Geometry check sheet. Reference: the model listing, model coordinates, mm. A direction names the side the tool comes from. Coordinates: 2 decimals unless noted, no trailing zeros. Loops run counter-clockwise (first coordinate to the right, second up) from the corner with the lowest first, then second, coordinate; pieces in that order, holes last. Notation, with made-up numbers: M -30.5,28 L 19.5,28 A29 cw 19.5,56 Z; hole C 44.25,-31 d7. An arc over 180 degrees is marked long. Use CSV: the item, a comma, the result in double quotes.
Autodesk Inventor part; units mm, degrees
ref_plane "YZ Plane" through (0, 0, 0) normal (1, 0, 0) x (0, 1, 0)
ref_plane "XZ Plane" through (0, 0, 0) normal (0, 1, 0) x (-1, 0, 0)
sketch "Sketch1" plane through (0, 0, 0) normal (1, 0, 0) x (0, 1, 0)
  line L0 (-5, 130) -> (-5, -130)
  line L1 (-5, -130) -> (5, -130)
  line L2 (5, -130) -> (5, 130)
  line L3 (5, 130) -> (-5, 130)
  line L4 (-5, 130) -> (5, -130) construction
  line L5 (-5, -130) -> (5, 130) construction
  circle A0 centre (0, -124) radius 1.95
  circle A1 centre (0, 124) radius 1.95
  line L6 (-5, -70) -> (-5, -60)
  circle A2 centre (0, -65) radius 1.5
  circle A3 centre (0, 65) radius 1.5
  point P0 (0, 0)
  point P1 (0, 0)
  dimension "d0" = 260
  dimension "d1" = 10
  dimension "d2" = 3.9
  dimension "d3" = 6
  dimension "d4" = 3.9
  dimension "d5" = 6
  dimension "d25" = 3
  dimension "d27" = 59
  dimension "d28" = 3
  dimension "d29" = 59
extrude "Extrusion1" add sketch "Sketch1" along normal blind 5
fillet "Fillet1" radius 2 4 edges at (2.5, 5, 130) (2.5, -5, 130) (2.5, 5, -130) (2.5, -5, -130)
sketch "Sketch2" plane through (5, 0, 0) normal (1, 0, 0) x (0, 0, -1)
  line L0 (-128, -5) -> (128, -5)
  line L1 (60, -5) -> (70, -5)
  line L2 (70, -5) -> (70, -25)
  line L3 (70, -25) -> (60, -25)
  line L4 (60, -25) -> (60, -5)
  circle A0 centre (65, -20) radius 1.5
  circle A1 centre (124, 0) radius 1.95
  line L5 (70, -25) -> (128, -5)
  line L6 (70, -19.7111) -> (112.6621, -5)
  point P0 (0, 0)
  dimension "d15" = 3
  dimension "d16" = 20
  dimension "d17" = 5
  dimension "d18" = 10
  dimension "d20" = 59
  dimension "d23" = 5
  dimension "d32" = 5
extrude "Extrusion2" add sketch "Sketch2" against normal blind 5 contours L0 L2 L3 L4 | L0 L5 L2 L6
mirror "Mirror1" about plane through (0, 0, 0) normal (0, 0, 1) of "Extrusion2"
sketch "Sketch4" plane through (5, 0, 0) normal (1, 0, 0) x (0, 0, -1)
  line L0 (-60, -25) -> (-60, -5)
  line L1 (60, -25) -> (60, -5)
  line L2 (-60, -25) -> (60, -25)
  line L3 (60, -25) -> (60, -20)
  line L4 (60, -20) -> (-60, -20)
  line L5 (-60, -20) -> (-60, -25)
  line L6 (-60, -25) -> (0, -5)
  line L7 (-60, -5) -> (60, -5)
  line L8 (70, -25) -> (60, -25)
  line L9 (0, -5) -> (60, -25)
  line L10 (60, -25) -> (60, -22.5)
  line L11 (6.3246, -5) -> (60, -22.8918)
  line L12 (-6.3246, -5) -> (-60, -22.8918)
  line L13 (-60, -5) -> (60, -5)
  line L14 (-1, -5) -> (1, -5)
  line L15 (1, -5) -> (1, -20)
  line L16 (1, -20) -> (-1, -20)
  line L17 (-1, -20) -> (-1, -5)
  point P0 (0, 0)
  point P1 (-60, -20)
  point P2 (-51.3246, -20)
  point P3 (-45, -20)
  point P4 (51.3246, -20)
  point P5 (45, -20)
  point P6 (-1, -5.3333)
  point P7 (-1, -20)
  point P8 (1, -5.3333)
  dimension "d33" = 5
  dimension "d37" = 2
  dimension "d38" = 2
  dimension "d39" = 1
  dimension "d40" = 1
extrude "Extrusion3" add sketch "Sketch4" against normal blind 5 contours L6 L4 L9 L2 | L0 L12 L4 L6 | L0 L4 L12 | L9 L4 L11 L1 | L4 L12 L7 L17 L6 | L11 L4 L1 | L9 L15 L7 L11 L4 | L17 L6 L9 L15 L4 | L17 L7 L6 | L9 L7 L15
fillet "Fillet3" radius 1 10 edges at (2.5, -19.7111, -70) (2.5, -5, -112.6621) (2.5, -5, -70) (2.5, -20, -60) (2.5, -5, -60) (2.5, -20, 60) (2.5, -5, 60) (2.5, -5, 112.6621) (2.5, -5, 70) (2.5, -19.7111, 70)
properties part number "Horizontal_bar"
1. Release check for a two-part mould opening along Y. For faces 3 (the flat face through (3, -25, -1)), 4 (the flat face through (3, -13, -60)), 5 (the flat face through (2, 0, 130)) record: +Y half, -Y half, draft (parallel to the pull), parting line (faces both ways), or undercut.
The answers:
face 3,"-Y half"
face 4,"undercut"
face 5,"draft"
2. Set-up check for faces 1 (the flat face through (3, -15, 99)), 2 (the flat face through (3, -13, -1)): record each of +Z, -Z, +X, -X, +Y, -Y from which the full face is reachable in a straight line by a thin tool's end or side.
The answers:
face 1,"+Z, +X, -X, -Y"
face 2,"+X, -X"
3. Section check C-C, the plane y = -14. Record the cut outline in (x, z), plus the area to 3 significant figures.
The answers:
outline,"M 0,-101.9 L 5,-101.9 L 5,-86.56 L 0,-86.56 Z; M 0,-70 L 5,-70 L 5,-60 L 0,-60 Z; M 0,-33.32 L 5,-33.32 L 5,-27 L 0,-27 Z; M 0,-1 L 5,-1 L 5,1 L 0,1 Z; M 0,27 L 5,27 L 5,33.32 L 0,33.32 Z; M 0,60 L 5,60 L 5,70 L 0,70 Z; M 0,86.56 L 5,86.56 L 5,101.9 L 0,101.9 Z"
area,"327 mm^2"
4. Section check B-B, the plane z = 23.5. Record the cut outline in (x, y).
The answers:
outline,"M 0,-25 L 5,-25 L 5,-20 L 0,-20 Z; M 0,-12.83 L 5,-12.83 L 5,-10.73 L 0,-10.73 Z; M 0,-5 L 5,-5 L 5,5 L 0,5 Z"
5. Thickness scan on line 1 (Z direction, x = 3.7, y = 0); line 2 (Y direction, x = 2.75, z = -65); line 3 (Y direction, x = 2.6, z = -10). Record the ranges inside material, lowest first. Write a range as [from, to].
The answers:
line 1,"[-130, -125.95], [-122.05, -66.5], [-63.5, 63.5], [66.5, 122.05], [125.95, 130]"
line 2,"[-25, -21.5], [-18.5, -1.5], [1.5, 5]"
line 3,"[-25, -20], [-8.33, -6.23], [-5, 5]"
6. Section check A-A, the plane z = 54. Record the cut outline in (x, y).
The answers:
outline,"M 0,-25 L 5,-25 L 5,-20 L 0,-20 Z; M 0,-5 L 5,-5 L 5,5 L 0,5 Z"
7. Section check D-D, the plane x = 0.95. Count the separate pieces of the cut face and the enclosed holes in it, plus the area to 3 significant figures.
The answers:
separate pieces,"1"
enclosed holes,"12"
area,"4,310 mm^2"
8. Gauge pin test, flat ends, axial feed: P1, Ø4, axis at y = -8, z = 94.5, coming from the -X side; P2, Ø1.5, axis at x = 3, z = 94.5, coming from the -Y side; P3, Ø2, axis at x = 4, z = -93.5, coming from the -Y side. Record the tip position at first contact, or that the pin passes through.
The answers:
P1,"through"
P2,"y = -16.81"
P3,"y = -17.24"
